Geometry check sheet. Reference: the model listing, model coordinates, mm. A direction names the side the tool comes from. Round coordinates to 2 decimals unless told otherwise and drop trailing zeros. Order: outer loops, then holes, each group sorted by start corner. A loop starts at its lowest first (then second) coordinate and runs counter-clockwise, first axis right, second up.
```python
from build123d import *

# Parameters (mm, degrees)
SKETCH1_R           = 3.25
BOSS_EXTRUDE1_DEPTH = 12.5
SKETCH2_R           = 1.75
CUT_EXTRUDE1_DEPTH  = 2.5
SKETCH6_R           = 4.8
BOSS_EXTRUDE2_DEPTH = 5
BOSS_EXTRUDE3_DEPTH = 1
FILLET1_R           = 0.75


with BuildPart() as part:
    # Sketch1 → Boss-Extrude1 (new body)
    with BuildSketch(Plane(origin=(0, 0, 0), x_dir=(1, 0, 0), z_dir=(0, 1, 0))):
        Circle(SKETCH1_R)
    extrude(amount=BOSS_EXTRUDE1_DEPTH)

    # Sketch2 → Cut-Extrude1 (cut)
    with BuildSketch(Plane.XZ):
        Circle(SKETCH2_R)
    extrude(amount=-CUT_EXTRUDE1_DEPTH, mode=Mode.SUBTRACT)

    # Sketch6 → Boss-Extrude2 (add)
    with BuildSketch(Plane(origin=(0, 12.5, 0), x_dir=(1, 0, 0), z_dir=(0, 1, 0))):
        Circle(SKETCH6_R)
    extrude(amount=BOSS_EXTRUDE2_DEPTH)

    # Sketch8 → Boss-Extrude3 (add)
    with BuildSketch(Plane(origin=(0, 17.5, 0), x_dir=(1, 0, 0), z_dir=(0, 1, 0))):
        Polygon((0.4, 3.75), (-0.4, 3.75), (-0.4, 0.4), (-3.75, 0.4), (-3.75, -0.4), (-0.4, -0.4), (-0.4, -3.75), (0.4, -3.75), (0.4, -0.4), (3.75, -0.4), (3.75, 0.4), (0.4, 0.4), align=None)
    extrude(amount=BOSS_EXTRUDE3_DEPTH)

    # Fillet1
    fillet1_edges = [part.edges().sort_by_distance(p)[0] for p in [
        (-4.8, 17.5, 0),
    ]]
    fillet(fillet1_edges, radius=FILLET1_R)


solid = part.part
```
(1) Material ranges on line 1 (Z direction, x = 0, y = 0.5); line 2 (Y direction, x = 0.75, z = 3); line 3 (X direction, y = 17.75, z = -2.75), recorded low to high.
Returned:
line 1: z = -3.25 to -1.75, 1.75 to 3.25
line 2: y = 0 to 17.5
line 3: x = -0.4 to 0.4
(2) Set-up check for faces 4 (the flat face through (-2, 18, 0.4)), 5 (the cylindrical face through (-2.579, 6.162, 1.978)), 6 (the flat face through (0.4, 18, 2)), 7 (the flat face through (-0.4, 18, -2)): record each of +Z, -Z, +X, -X, +Y, -Y from which the full face is reachable in a straight line by a thin tool's end or side.
Returned:
face 4: +Z, -X, +Y
face 5: -Y
face 6: +Z, +X, +Y
face 7: -Z, -X, +Y
(3) Depth check by flat-ended pin: P1, Ø0.8, axis at x = -1, y = 18, coming from the -Z side; P2, Ø1, axis at x = -1, z = -2, coming from the +Y side; P3, Ø2, axis at x = -1.5, y = 4, coming from the -Z side; P4, Ø3, axis at x = 0.5, z = -0.5, coming from the -Y side. Enter the tip coordinate at first touch or a pass-through.
Returned:
P1: stops at z = -0.4
P2: stops at y = 17.5
P3: stops at z = -3.21
P4: stops at y = 0
(4) Sectioned sample at B-B, the plane x = 0. Record the cut outline in (y, z), and give its area (3 significant figures).
Returned:
outline: (0, -3.25) - (12.5, -3.25) - (12.5, -4.8) - (16.75, -4.8) arc R0.75 ccw to (17.5, -4.05) - (17.5, -3.75) - (18.5, -3.75) - (18.5, 3.75) - (17.5, 3.75) - (17.5, 4.05) arc R0.75 ccw to (16.75, 4.8) - (12.5, 4.8) - (12.5, 3.25) - (0, 3.25) - (0, 1.75) - (2.5, 1.75) - (2.5, -1.75) - (0, -1.75) - close
area: 128 mm2
(5) Sectioned sample at A-A, the plane y = 1.75. Record the cut outline in (x, z).
Returned:
outline: circle Ø6.5 at (0, 0); hole circle Ø3.5 at (0, 0)
(6) Sectioned sample at C-C, the plane z = 0. Record the cut outline in (x, y).
Returned:
outline: (-4.8, 12.5) - (-3.25, 12.5) - (-3.25, 0) - (-1.75, 0) - (-1.75, 2.5) - (1.75, 2.5) - (1.75, 0) - (3.25, 0) - (3.25, 12.5) - (4.8, 12.5) - (4.8, 16.75) arc R0.75 ccw to (4.05, 17.5) - (3.75, 17.5) - (3.75, 18.5) - (-3.75, 18.5) - (-3.75, 17.5) - (-4.05, 17.5) arc R0.75 ccw to (-4.8, 16.75) - close
(7) Sectioned sample at D-D, the plane y = 9.25. Record the cut outline in (x, z), and give its area (3 significant figures).
Returned:
outline: circle Ø6.5 at (0, 0)
area: 33.2 mm2
(8) Draft check along Z on faces 1 (the flat face through (2, 18, -0.4)), 2 (the flat face through (-0.4, 18, 2)), 3 (the flat face through (0, 2.5, 0)). Enter one of: released by +Z, released by -Z, zero draft, split by the parting line, or undercut.
Returned:
face 1: released by -Z
face 2: zero draft
face 3: undercut
